```python
from build123d import *

# Parameters (mm, degrees)
F0_W     = 254
F0_H     = 152.4
F1_DEPTH = 3.4036


# Not quite as in the source:
# - a feature names something its author has since deleted; it is built from what else it names


with BuildPart() as f1:
    # F0 (on Front) → F1 (new body)
    with BuildSketch(Plane.XZ):
        Polygon((196.4755472482, 406.4), (0, 0), (914.4, 0), (704.4755472482, 406.4), align=None)
        with Locations((450.4755472482, 203.2)):
            Rectangle(F0_W, F0_H, mode=Mode.SUBTRACT)
    extrude(amount=F1_DEPTH)


solid = f1.part
```
For this review, take the finished solid that the model builds, in its own axes (mm). Round coordinates to 2 decimals unless told otherwise and drop trailing zeros. Write each loop counter-clockwise with the first axis right and the second up, starting at its lowest first coordinate (ties: lowest second). Pieces come first, ordered by that corner, then holes. Notation, with made-up numbers: (16, 89) - (48, 89) arc R13 ccw to (48, 97) - close; hole circle Ø11 at (82, 28). An arc over 180 degrees is marked (long way). Put each result on its own line as item: value.
Q1. We need section A-A (x = 364.5). Give the boundary of the cut face in (y, z), and give its area (3 significant figures).
Solved:
outline: (-3.4, 0) - (0, 0) - (0, 127) - (-3.4, 127) - close; (-3.4, 279.4) - (0, 279.4) - (0, 406.4) - (-3.4, 406.4) - close
area: 865 mm2
Q2. We need section B-B (z = 211). Give the boundary of the cut face in (x, y), and give its area (3 significant figures).
Solved:
outline: (102.01, -3.4) - (323.48, -3.4) - (323.48, 0) - (102.01, 0) - close; (577.48, -3.4) - (805.41, -3.4) - (805.41, 0) - (577.48, 0) - close
area: 1,530 mm2
Q3. Insertion check: pin 1 Ø1 at (y, z) = (-2, 228) entering from -X; pin 2 Ø1.7 at (y, z) = (-2, 176.5) entering from +X; pin 3 Ø1 at (x, y) = (117.5, -2.5) entering from +Z. Each pin has a flat end and moves straight along its axis. Give the tip position at first contact, or say it passes through.
Solved:
pin 1: stops at x = 109.99
pin 2: stops at x = 823.67
pin 3: stops at z = 244.08
Q4. Wall thickness on probe 1 along Z at (x, y) = (560, -2.2); probe 2 along X at (y, z) = (-0.85, 242.5); probe 3 along X at (y, z) = (-1.1, 269.5): over which ranges is each line inside the solid? List them lowest first.
Solved:
probe 1: z = 0 to 127, 279.4 to 406.4
probe 2: x = 117.24 to 323.48, 577.48 to 789.14
probe 3: x = 130.29 to 323.48, 577.48 to 775.19
Q5. We need section C-C (y = -2.05). Give the boundary of the cut face in (x, z), and give its area (3 significant figures).
Solved:
outline: (0, 0) - (914.4, 0) - (704.48, 406.4) - (196.48, 406.4) - close; hole (323.48, 127) - (577.48, 127) - (577.48, 279.4) - (323.48, 279.4) - close
area: 250,000 mm2
Q6. We need section D-D (x = 183). Give the boundary of the cut face in (y, z), and give its area (3 significant figures).
Solved:
outline: (-3.4, 0) - (0, 0) - (0, 378.53) - (-3.4, 378.53) - close
area: 1,290 mm2
